The drawing under review shows one solid part. Ordinate dimensions are in mm from its lowest x, y, z. Round coordinates to 2 decimals unless told otherwise and drop trailing zeros. Order: outer loops, then holes, each group sorted by start corner. A loop starts at its lowest first (then second) coordinate and runs counter-clockwise, first axis right, second up. Notation, with made-up numbers: M 28,19.25 L 58,19.25 A23 ccw 58,51.25 Z; hole C -21.5,64 d7. An arc over 180 degrees is marked long. Answer in a Markdown table with one row per item. Add a question column.
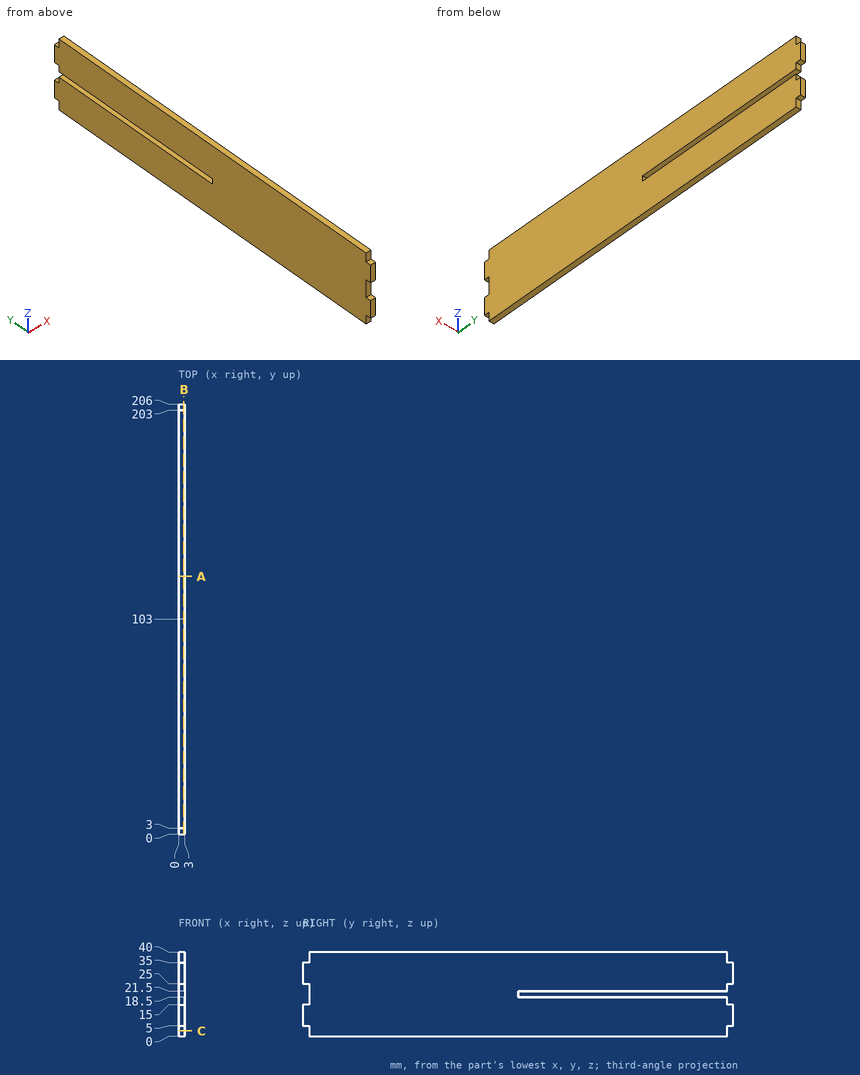
1. Consider section B-B on x = 2.55. Write out the cut boundary in (y, z), plus the area to 3 significant figures.
2. To check wall thickness, follow probe 1 along Z at (x, y) = (2.4, 131); probe 2 along Y at (x, z) = (2.85, 22). State the ranges of each line that lie inside material, in increasing order. Write a range as [from, to].
3. Consider section C-C on z = 2.5. Write out the cut boundary in (x, y), plus the area to 3 significant figures.
4. Clearance check with flat-ended pins moving along their axes: pin 1 Ø1.5 at (x, y) = (1.5, 204) entering from +Z; pin 2 Ø0.9 at (x, z) = (1, 20.5) entering from +Y; pin 3 Ø0.9 at (x, y) = (1.5, 1) entering from -Z. State where each tip first meets the part, or that it passes through.
5. Consider section A-A on y = 123.5. Write out the cut boundary in (x, z).
Solved:
| question | item | result |
|---|---|---|
| 1 | outline | M 0,5 L 3,5 L 3,0 L 203,0 L 203,5 L 206,5 L 206,15 L 203,15 L 203,18.5 L 103,18.5 L 103,21.5 L 203,21.5 L 203,25 L 206,25 L 206,35 L 203,35 L 203,40 L 3,40 L 3,35 L 0,35 L 0,25 L 3,25 L 3,15 L 0,15 Z |
| 1 | area | 7,820 mm^2 |
| 2 | probe 1 | z = [0, 18.5], [21.5, 40] |
| 2 | probe 2 | y = [3, 203] |
| 3 | outline | M 0,3 L 3,3 L 3,203 L 0,203 Z |
| 3 | area | 600 mm^2 |
| 4 | pin 1 | stops at z = 35 |
| 4 | pin 2 | stops at y = 103 |
| 4 | pin 3 | stops at z = 5 |
| 5 | outline | M 0,0 L 3,0 L 3,18.5 L 0,18.5 Z; M 0,21.5 L 3,21.5 L 3,40 L 0,40 Z |
